from build123d import *

# Parameters (mm, degrees)
SKETCH_1_W          = 200
SKETCH_1_H          = 200
EXTRUDE_1_DEPTH     = 4
SKETCH_2_W          = 2
SKETCH_2_H          = 200
EXTRUDE_2_DEPTH     = 20
SKETCH_4_R          = 3.25
SKETCH_4_R_2        = 1.6
CUT_EXTRUDE_1_DEPTH = 10
SKETCH_5_W          = 21
SKETCH_5_H          = 25
EXTRUDE_3_DEPTH     = 5


with BuildPart() as part:
    # 草图1 → 凸台-拉伸1 (new body)
    with BuildSketch(Plane(origin=(0, 0, 0), x_dir=(1, 0, 0), z_dir=(0, 1, 0))):
        Rectangle(SKETCH_1_W, SKETCH_1_H)
    extrude(amount=EXTRUDE_1_DEPTH)

    # 草图2 → 凸台-拉伸2 (add)
    with BuildSketch(Plane.XZ):
        with Locations((-69, 0)):
            Rectangle(SKETCH_2_W, SKETCH_2_H)
        with Locations((-92, 0)):
            Rectangle(SKETCH_2_W, SKETCH_2_H)
    extrude_2 = extrude(amount=EXTRUDE_2_DEPTH)

    # 镜向1: 凸台-拉伸2 across plane
    add(extrude_2.mirror(Plane(origin=(0, 0, 0), x_dir=(0, 0, 1), z_dir=(1, 0, 0))))

    # 草图4 → 切除-拉伸1 (cut)
    with BuildSketch(Plane(origin=(0, 4, 0), x_dir=(1, 0, 0), z_dir=(0, 1, 0))):
        with Locations(Location((18.5, 18.5, 0), (0, 0, 270))):
            Circle(SKETCH_4_R)
        with Locations(Location((18.5, -18.5, 0), (0, 0, 270))):
            Circle(SKETCH_4_R)
        with Locations(Location((-18.5, -18.5, 0), (0, 0, 270))):
            Circle(SKETCH_4_R)
        with Locations(Location((-18.5, 18.5, 0), (0, 0, 270))):
            Circle(SKETCH_4_R)
        with Locations(Location((97, -50, 0), (0, 0, 270))):
            Circle(SKETCH_4_R_2)
        with Locations(Location((97, 50, 0), (0, 0, 270))):
            Circle(SKETCH_4_R_2)
        with Locations(Location((-97, -50, 0), (0, 0, 270))):
            Circle(SKETCH_4_R_2)
        with Locations(Location((-97, 50, 0), (0, 0, 270))):
            Circle(SKETCH_4_R_2)
        with Locations(Location((-97, 0, 0), (0, 0, 270))):
            Circle(SKETCH_4_R_2)
        with Locations(Location((97, 0, 0), (0, 0, 270))):
            Circle(SKETCH_4_R_2)
    extrude(amount=-CUT_EXTRUDE_1_DEPTH, mode=Mode.SUBTRACT)

    # 草图5 → 凸台-拉伸3 (add)
    with BuildSketch(Plane.XZ):
        with Locations((80.5, 87.5)):
            Rectangle(SKETCH_5_W, SKETCH_5_H)
        with Locations((80.5, -87.5)):
            Rectangle(SKETCH_5_W, SKETCH_5_H)
    extrude_3 = extrude(amount=EXTRUDE_3_DEPTH)

    # 镜向2: 凸台-拉伸3 across plane
    add(extrude_3.mirror(Plane(origin=(0, 0, 0), x_dir=(0, 0, 1), z_dir=(1, 0, 0))))


solid = part.part
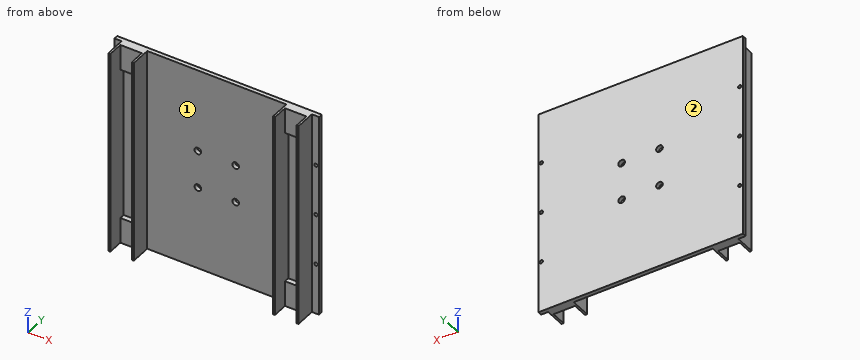
Can you work these out from the model? Positions are in its coordinate system, mm. Face numbers are marked on the shaded views. Coordinates: 2 decimals unless noted, no trailing zeros. Write each loop counter-clockwise with the first axis right and the second up, starting at its lowest first coordinate (ties: lowest second). Pieces come first, ordered by that corner, then holes. Notation, with made-up numbers: (62.5, 17) - (93.5, 17) arc R6 cw to (93.5, 25) - close; hole circle Ø5 at (65.25, 7.25). An arc over 180 degrees is marked (long way). Return JSON: item names as keys, results as strings. Group by question number.
Item 1: Please list where these lines run through material, in increasing order: probe 1 along X at (y, z) = (-8.5, 36.5); probe 2 along Z at (x, y) = (97, 3.15); probe 3 along X at (y, z) = (2.55, 50).
Item 2: If we section it at C-C (y = -10.75): Write out the boundary of the cut face in (x, z), then the cut area to 3 significant figures.
Item 3: We'd pull the mould along X, two halves only. Please class the marked faces 1 and 2: pulls with the +X half, pulls with the -X half, needs draft (parallel to the pull), parting line crosses it, or undercut.
Item 4: If we section it at A-A (z = -18.5): Write out the boundary of the cut face in (x, y), then the cut area to 3 significant figures.
Item 5: If we section it at D-D (z = -87.5): Write out the boundary of the cut face in (x, y), then the cut area to 3 significant figures.
Item 6: I'm going to push flat-ended pins straight in: pin 1 Ø5 at (x, z) = (-97, 0) entering from -Y; pin 2 Ø1 at (y, z) = (-14.5, 75) entering from +X; pin 3 Ø8.5 at (x, z) = (18.5, 18.5) entering from +Y; pin 4 Ø6 at (y, z) = (-14.5, 4) entering from -X. Where does each tip first touch, or does it pass through?
Item 7: If we section it at B-B (x = -18.5): Write out the boundary of the cut face in (y, z), then the cut area to 3 significant figures.
Return value:
{
 "1": {"probe 1": "x = -93 to -91, -70 to -68, 68 to 70, 91 to 93", "probe 2": "z = -100 to -51.6, -48.4 to -1.6, 1.6 to 48.4, 51.6 to 100", "probe 3": "x = -100 to -98.6, -95.4 to 95.4, 98.6 to 100"},
 "2": {"outline": "(-93, -100) - (-91, -100) - (-91, 100) - (-93, 100) - close; (-70, -100) - (-68, -100) - (-68, 100) - (-70, 100) - close; (68, -100) - (70, -100) - (70, 100) - (68, 100) - close; (91, -100) - (93, -100) - (93, 100) - (91, 100) - close", "area": "1,600 mm^2"},
 "3": {"face 1": "undercut", "face 2": "needs draft"},
 "4": {"outline": "(-100, 0) - (-93, 0) - (-93, -20) - (-91, -20) - (-91, 0) - (-70, 0) - (-70, -20) - (-68, -20) - (-68, 0) - (-21.75, 0) - (-21.75, 4) - (-100, 4) - close; (-15.25, 0) - (15.25, 0) - (15.25, 4) - (-15.25, 4) - close; (21.75, 0) - (68, 0) - (68, -20) - (70, -20) - (70, 0) - (91, 0) - (91, -20) - (93, -20) - (93, 0) - (100, 0) - (100, 4) - (21.75, 4) - close", "area": "908 mm^2"},
 "5": {"outline": "(-100, 0) - (-93, 0) - (-93, -20) - (-91, -20) - (-91, -5) - (-70, -5) - (-70, -20) - (-68, -20) - (-68, 0) - (68, 0) - (68, -20) - (70, -20) - (70, -5) - (91, -5) - (91, -20) - (93, -20) - (93, 0) - (100, 0) - (100, 4) - (-100, 4) - close", "area": "1,170 mm^2"},
 "6": {"pin 1": "stops at y = 0", "pin 2": "stops at x = 93", "pin 3": "stops at y = 4", "pin 4": "stops at x = -93"},
 "7": {"outline": "(0, -100) - (4, -100) - (4, -21.75) - (0, -21.75) - close; (0, -15.25) - (4, -15.25) - (4, 15.25) - (0, 15.25) - close; (0, 21.75) - (4, 21.75) - (4, 100) - (0, 100) - close", "area": "748 mm^2"}
}
